Input: part model. Units: mm. Frame: model coordinates. A direction names the side the tool comes from. Coordinates: 2 decimals unless noted, no trailing zeros. Order: outer loops, then holes, each group sorted by start corner. A loop starts at its lowest first (then second) coordinate and runs counter-clockwise, first axis right, second up. Notation, with made-up numbers: (36, 77) -> (49, 77) arc R16 cw to (49, 105) -> close; hole circle Ø7 at (24.25, 7.25). An arc over 180 degrees is marked (long way). One line per question, with ' | ' between items.
Autodesk Inventor part; units mm, degrees
ref_plane "Work Plane2" through (0, 0, 10) normal (0, 0, 1) x (1, 0, 0)
ref_plane "Work Plane8" through (0, 0, 0) normal (0.9396926, 0.3420201, 0) x (0, 0, 1)
ref_plane "Work Plane9" through (0, 0, 0) normal (1, 0, 0) x (0, 1, 0)
sketch "Sketch1" plane through (0, 0, 0) normal (0, 0, 1) x (1, 0, 0)
  circle A0 centre (0, 0) radius 5.5
  dimension "d0" = 11
extrude "Extrusion1" add sketch "Sketch1" along normal blind 20
ref_plane "Work Plane2" through (0, 0, 10) normal (0, 0, 1) x (1, 0, 0)
sketch "Sketch2" plane through (0, 0, 0) normal (0, 0, -1) x (-1, 0, 0)
  circle A0 centre (0, 0) radius 5.5
  circle A1 centre (0, 0) radius 4.5
  dimension "d3" = 9
surface extrude "ピッチ円直径" sketch "Sketch2" against normal through all shown no curves A1
ref_plane "Work Plane8" through (0, 0, 0) normal (0.9396926, 0.3420201, 0) x (0, 0, 1)
ref_plane "Work Plane9" through (0, 0, 0) normal (1, 0, 0) x (0, 1, 0)
spur gear teeth "平歯車" teeth 9 pitch diameter 9 tip diameter 11 root diameter 6.5 face width 20 start plane through (0, 0, 0) normal (0, 0, -1) x (-1, 0, 0)
sketch "スケッチ3" plane through (0, 0, 20) normal (0, 0, 1) x (1, 0, 0)
  arc A0 (-3.8891, 3.8891) -> (-2.6622, 1.8641) centre (0.9613, 5.4436) ccw
  arc A1 (-2.6622, 1.8641) -> (-2.9455, 1.3735) centre (0, 0) ccw
  arc A2 (-2.9455, 1.3735) -> (-5.3126, 1.4235) centre (-4.2337, -3.5543) ccw
  arc A3 (-5.3126, 1.4235) -> (-5.4791, 0.4794) centre (0, 0) ccw
  arc A4 (-5.4791, 0.4794) -> (-3.2376, -0.2833) centre (-2.7627, 4.7879) ccw
  arc A5 (-3.2376, -0.2833) -> (-3.1393, -0.8412) centre (0, 0) ccw
  arc A6 (-3.1393, -0.8412) -> (-4.9847, -2.3244) centre (-0.9585, -5.4441) ccw
  arc A7 (-4.9847, -2.3244) -> (-4.5053, -3.1547) centre (0, 0) ccw
  arc A8 (-4.5053, -3.1547) -> (-2.2981, -2.2981) centre (-5.194, 1.8919) ccw
  arc A9 (-2.2981, -2.2981) -> (-1.8641, -2.6622) centre (0, 0) ccw
  arc A10 (-1.8641, -2.6622) -> (-2.3244, -4.9847) centre (2.7651, -4.7865) ccw
  arc A11 (-2.3244, -4.9847) -> (-1.4235, -5.3126) centre (0, 0) ccw
  arc A12 (-1.4235, -5.3126) -> (-0.2833, -3.2376) centre (-5.1949, -1.8893) ccw
  arc A13 (-0.2833, -3.2376) -> (0.2833, -3.2376) centre (0, 0) ccw
  arc A14 (0.2833, -3.2376) -> (1.4235, -5.3126) centre (5.1949, -1.8893) ccw
  arc A15 (1.4235, -5.3126) -> (2.3244, -4.9847) centre (0, 0) ccw
  arc A16 (2.3244, -4.9847) -> (1.8641, -2.6622) centre (-2.7651, -4.7865) ccw
  arc A17 (1.8641, -2.6622) -> (2.2981, -2.2981) centre (0, 0) ccw
  arc A18 (2.2981, -2.2981) -> (4.5053, -3.1547) centre (5.194, 1.8919) ccw
  arc A19 (4.5053, -3.1547) -> (4.9847, -2.3244) centre (0, 0) ccw
  arc A20 (4.9847, -2.3244) -> (3.1393, -0.8412) centre (0.9585, -5.4441) ccw
  arc A21 (3.1393, -0.8412) -> (3.2376, -0.2833) centre (0, 0) ccw
  arc A22 (3.2376, -0.2833) -> (5.4791, 0.4794) centre (2.7627, 4.7879) ccw
  arc A23 (5.4791, 0.4794) -> (5.3126, 1.4235) centre (0, 0) ccw
  arc A24 (5.3126, 1.4235) -> (2.9455, 1.3735) centre (4.2337, -3.5543) ccw
  arc A25 (2.9455, 1.3735) -> (2.6622, 1.8641) centre (0, 0) ccw
  arc A26 (2.6622, 1.8641) -> (3.8891, 3.8891) centre (-0.9613, 5.4436) ccw
  arc A27 (3.8891, 3.8891) -> (3.1547, 4.5053) centre (0, 0) ccw
  arc A28 (3.1547, 4.5053) -> (1.3735, 2.9455) centre (5.5278, -0.0014) ccw
  arc A29 (1.3735, 2.9455) -> (0.8412, 3.1393) centre (0, 0) ccw
  arc A30 (0.8412, 3.1393) -> (0.4794, 5.4791) centre (-4.2354, 3.5521) ccw
  arc A31 (0.4794, 5.4791) -> (-0.4794, 5.4791) centre (0, 0) ccw
  arc A32 (-0.4794, 5.4791) -> (-0.8412, 3.1393) centre (4.2354, 3.5521) ccw
  arc A33 (-0.8412, 3.1393) -> (-1.3735, 2.9455) centre (0, 0) ccw
  arc A34 (-1.3735, 2.9455) -> (-3.1547, 4.5053) centre (-5.5278, -0.0014) ccw
  arc A35 (-3.1547, 4.5053) -> (-3.8891, 3.8891) centre (0, 0) ccw
equation "\"d0\" = da_da"
equation "\"d1\" = da_b"
equation "\"d3\" = da_dw"
properties part number "平歯車1" material "Steel"
1. Cut plane D-D, the plane y = -1.25. Return loops of the section in (x, z), and give its area (3 significant figures).
Recorded:
outline: (-3.85, 0) -> (3.85, 0) -> (3.85, 20) -> (-3.85, 20) -> close | area: 154 mm^2
2. Mould query, pull axis X, two halves, no side actions, for faces 4 (the face through (-3.34, -2.85, 9.86)), 5 (the face through (-5.418, 0.948, 9.86)), 6 (the face through (0, 0, 0)). Classes: released by +X, released by -X, zero draft, split by the parting line, or undercut.
Recorded:
face 4: undercut | face 5: released by -X | face 6: zero draft
3. Access query for faces 1 (the face through (-4.39, -0.04, 9.86)), 2 (the face through (3.404, 2.819, 9.86)), 3 (the face through (-4.14, 1.54, 9.86)). Directions: +Z, -Z, +X, -X, +Y, -Y. A direction counts if a zero-diameter tool reaches every point of the face in a straight line with its end or side. Return the directions, or none.
Recorded:
face 1: +Z, -Z, -X | face 2: +Z, -Z, +X | face 3: +Z, -Z
4. Cut plane B-B, the plane x = 3.5. Return loops of the section in (y, z).
Recorded:
outline: (-2.91, 0) -> (-1.03, 0) -> (-1.03, 20) -> (-2.91, 20) -> close; (-0.25, 0) -> (1.49, 0) -> (1.49, 20) -> (-0.25, 20) -> close; (2.99, 0) -> (4.24, 0) -> (4.24, 20) -> (2.99, 20) -> close
5. Cut plane A-A, the plane y = -3.75. Return loops of the section in (x, z).
Recorded:
outline: (-2.22, 0) -> (-0.45, 0) -> (-0.45, 20) -> (-2.22, 20) -> close; (0.45, 0) -> (2.22, 0) -> (2.22, 20) -> (0.45, 20) -> close
6. Ray query, line 1 (Y direction, x = 3.5, z = 10.25); line 2 (Y direction, x = -3.75, z = 17.25); line 3 (Y direction, x = 4, z = 6.25). Return the intervals inside material, ascending. Write a range as [from, to].
Recorded:
line 1: y = [-2.91, -1.03], [-0.25, 1.49], [2.99, 4.24] | line 2: y = [-2.99, -1.18], [-0.21, 1.52], [3.51, 4.02] | line 3: y = [-3.06, -1.36], [-0.15, 1.53]
7. Cut plane C-C, the plane x = 0. Return loops of the section in (y, z), and give its area (3 significant figures).
Recorded:
outline: (-3.25, 0) -> (5.5, 0) -> (5.5, 20) -> (-3.25, 20) -> close | area: 175 mm^2
8. Pin query (flat end, axial travel): pin 1 Ø5 at (y, z) = (3, 8) entering from +X; pin 2 Ø6 at (y, z) = (-3.5, 4) entering from -X. Return the tip coordinate at first contact, or that it passes through.
Recorded:
pin 1: stops at x = 5.48 | pin 2: stops at x = -4.98
